Verification items for the finished model (mm, model axes). Face numbers are marked on the shaded views. A direction names the side the tool comes from. Round coordinates to 2 decimals unless told otherwise and drop trailing zeros. Order: outer loops, then holes, each group sorted by start corner. A loop starts at its lowest first (then second) coordinate and runs counter-clockwise, first axis right, second up. Notation, with made-up numbers: M 82.5,19.25 L 111.5,19.25 A7 cw 111.5,24.25 Z; hole C 47,82.25 d5. An arc over 180 degrees is marked long. Write item = value, one per line. Start each with the question number.
from build123d import *

# Parameters (mm, degrees)
F0_W     = 40
F0_H     = 76
F0_R     = 1.75
F1_DEPTH = 44
F2_W     = 72
F2_H     = 40
F3_DEPTH = 36
F4_R     = 1.5
F5_DEPTH = 4
F6_DEPTH = 4
F7_R     = 3.99999


# Not quite as in the source:
# - a fillet or chamfer is up to 0.001 mm smaller than in the source, because OpenCascade refuses the exact size


with BuildPart() as f1:
    # F0 (on Top) → F1 (new body)
    with BuildSketch(Plane.XY):
        with Locations((20, 38)):
            Rectangle(F0_W, F0_H)
        with Locations((10, 16.5)):
            Circle(F0_R, mode=Mode.SUBTRACT)
        with Locations((10, 63.5)):
            Circle(F0_R, mode=Mode.SUBTRACT)
        with Locations((10, 63.5)):
            Circle(F0_R)
        with Locations((10, 16.5)):
            Circle(F0_R)
    extrude(amount=F1_DEPTH)

    # F2 (on face) → F3 (cut)
    with BuildSketch(Plane(origin=(0, 0, 0), x_dir=(0, -1, 0), z_dir=(-1, 0, 0))):
        with Locations((-40, 24)):
            Rectangle(F2_W, F2_H)
    extrude(amount=-F3_DEPTH, mode=Mode.SUBTRACT)

    # F4 (on face) → F5 (cut)
    with BuildSketch(Plane(origin=(0, 76, 0), x_dir=(-1, 0, 0), z_dir=(0, 1, 0))):
        with BuildLine():
            ThreePointArc((-29.5, 18.5), (-26.6715728753, 19.6715728753), (-25.5, 22.5))
            ThreePointArc((-25.5, 22.5), (-26.6715728753, 25.3284271247), (-29.5, 26.5))
            ThreePointArc((-29.5, 26.5), (-33.5, 22.5), (-29.5, 18.5))
        make_face()
        with Locations((-12, 23.5)):
            Circle(F4_R)
    extrude(amount=-F5_DEPTH, mode=Mode.SUBTRACT)

    # F0 (on Top) → F6 (cut)
    with BuildSketch(Plane.XY):
        with Locations((10, 63.5)):
            Circle(F0_R)
        with Locations((10, 16.5)):
            Circle(F0_R)
    extrude(amount=F6_DEPTH, mode=Mode.SUBTRACT)

    # F7 (radius 4 in the source; OpenCascade refuses exactly that, so slightly less here)
    f7_edges = [f1.edges().sort_by_distance(p)[0] for p in [
        (40, 38, 0),
        (40, 0, 22),
        (0, 0, 22),
        (20, 0, 0),
        (0, 76, 2),
        (0, 38, 0),
    ]]
    fillet(f7_edges, radius=F7_R)


solid = f1.part
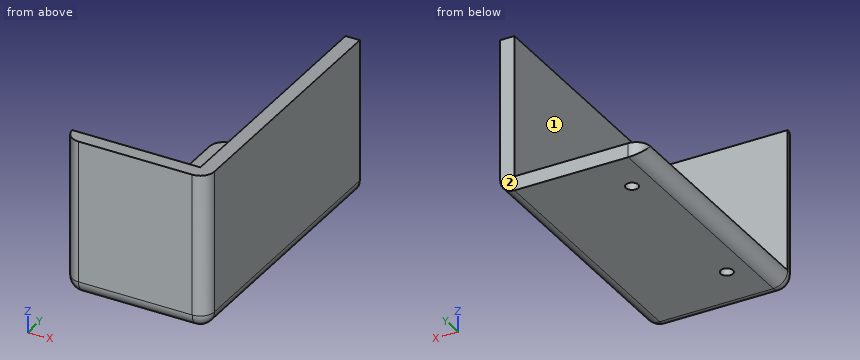
1) Cross-section at B-B, the plane x = 10.5. Enter the section's corners in (y, z), then the cut area to 3 significant figures.
2) Gauge pin test, flat ends, axial feed: P1, Ø20, axis at y = 40.5, z = 16.5, coming from the -X side; P2, Ø18, axis at x = 23, y = 57, coming from the +Z side. Record the tip position at first contact, or that the pin passes through.
3) Access from +Z, -Z, +X, -X, +Y, -Y to the whole of each face (thin tool, end or side, straight path). Record for the marked faces 1 and 2.
4) Scan lines: probe 1 along Y at (x, z) = (10, 1.3); probe 2 along Y at (x, z) = (10, 2); probe 3 along X at (y, z) = (63.5, 28.5). Record each from-to range of solid material in increasing order.
Geometry results:
q1.outline = M 0,4 A4 ccw 4,0 L 14.82,0 L 14.82,4 L 4,4 L 4,44 L 0,44 Z; M 18.18,0 L 61.82,0 L 61.82,4 L 18.18,4 Z; M 65.18,0 L 76,0 L 76,4 L 65.18,4 Z
q1.area = 434 mm^2
q2.P1 = 36
q2.P2 = 4
q3.face_1 = +Z, -X, +Y
q3.face_2 = +Z, -Z, +X, -X, +Y
q4.probe_1 = 1.05 to 14.75, 18.25 to 61.75, 65.25 to 76
q4.probe_2 = 0.54 to 14.75, 18.25 to 61.75, 65.25 to 76
q4.probe_3 = 36 to 40
